Geometry: final body of the model. Coordinates: model frame, mm. A direction names the side the tool comes from. Give positions to 0.01 mm unless a question says otherwise; leave off trailing zeros. Loops run counter-clockwise (first coordinate to the right, second up) from the corner with the lowest first, then second, coordinate; pieces in that order, holes last. Notation, with made-up numbers: (-1, 48) - (22, 48) arc R30 cw to (22, 78) - close; hole circle Ø6 at (21, 56). An arc over 180 degrees is marked (long way). Use CSV: the item, a comma, the result in double quotes. Start each with the question number.
```python
from build123d import *

# Parameters (mm, degrees)
ESBO_O1_R                = 1.5
ESBO_O1_W                = 5
ESBO_O1_H                = 35
RESSALTO_EXTRUS_O1_DEPTH = 3
ESBO_O2_W                = 25
ESBO_O2_H                = 5
RESSALTO_EXTRUS_O2_DEPTH = 15
FILETE5_R                = 5
FILETE6_R                = 5
FILETE7_R                = 5
FILETE8_R                = 5
ESBO_O4_R                = 1
ESBO_O4_W                = 4
ESBO_O4_H                = 4
CORTE_EXTRUS_O2_DEPTH    = 5
CORTE_EXTRUS_O3_START    = -5
ESBO_O3_R                = 1
ESBO_O3_R_2              = 1.5
ESBO_O3_W                = 4
ESBO_O3_H                = 7
CORTE_EXTRUS_O3_DEPTH    = 5


with BuildPart() as part:
    # Esboço1 → Ressalto-extrusão1 (new body)
    with BuildSketch(Plane.XY):
        Polygon((-24.430369357, 7.066666667), (10.569630643, 7.066666667), (10.569630643, 2.066666667), (5.569630643, 2.066666667), (5.569630643, -32.933333333), (10.569630643, -32.933333333), (10.569630643, -37.933333333), (-24.430369357, -37.933333333), (-24.430369357, -32.933333333), (-19.430369357, -32.933333333), (-19.430369357, 2.066666667), (-24.430369357, 2.066666667), align=None)
        with Locations((-14.430369357, -4.933333333)):
            Circle(ESBO_O1_R, mode=Mode.SUBTRACT)
        with Locations((-14.430369357, -11.933333333)):
            Circle(ESBO_O1_R, mode=Mode.SUBTRACT)
        with Locations((-14.430369357, -18.933333333)):
            Circle(ESBO_O1_R, mode=Mode.SUBTRACT)
        with Locations((0.569630643, -4.933333333)):
            Circle(ESBO_O1_R, mode=Mode.SUBTRACT)
        with Locations((0.569630643, -18.933333333)):
            Circle(ESBO_O1_R, mode=Mode.SUBTRACT)
        with Locations((0.569630643, -25.933333333)):
            Circle(ESBO_O1_R, mode=Mode.SUBTRACT)
        with Locations((-14.430369357, -25.933333333)):
            Circle(ESBO_O1_R, mode=Mode.SUBTRACT)
        with Locations((0.569630643, -11.933333333)):
            Circle(ESBO_O1_R, mode=Mode.SUBTRACT)
        with Locations((-21.930369357, 4.566666667)):
            Circle(ESBO_O1_R, mode=Mode.SUBTRACT)
        with Locations((8.069630643, 4.566666667)):
            Circle(ESBO_O1_R, mode=Mode.SUBTRACT)
        with Locations((-21.930369357, -35.433333333)):
            Circle(ESBO_O1_R, mode=Mode.SUBTRACT)
        with Locations((8.069630643, -35.433333333)):
            Circle(ESBO_O1_R, mode=Mode.SUBTRACT)
        with Locations((-6.930369357, -15.433333333)):
            Rectangle(ESBO_O1_W, ESBO_O1_H, mode=Mode.SUBTRACT)
    extrude(amount=-RESSALTO_EXTRUS_O1_DEPTH)

    # Esboço2 → Ressalto-extrusão2 (add)
    with BuildSketch(Plane.XY):
        with Locations((-6.930369357, 4.566666667)):
            Rectangle(ESBO_O2_W, ESBO_O2_H)
        with Locations((-6.930369357, -35.433333333)):
            Rectangle(ESBO_O2_W, ESBO_O2_H)
    extrude(amount=RESSALTO_EXTRUS_O2_DEPTH)

    # Filete5
    filete5_edges = [part.edges().sort_by_distance(p)[0] for p in [
        (5.569630643, -35.433333333, 15),
    ]]
    fillet(filete5_edges, radius=FILETE5_R)

    # Filete6
    filete6_edges = [part.edges().sort_by_distance(p)[0] for p in [
        (-19.430369357, -35.433333333, 15),
    ]]
    fillet(filete6_edges, radius=FILETE6_R)

    # Filete7
    filete7_edges = [part.edges().sort_by_distance(p)[0] for p in [
        (-19.430369357, 4.566666667, 15),
    ]]
    fillet(filete7_edges, radius=FILETE7_R)

    # Filete8
    filete8_edges = [part.edges().sort_by_distance(p)[0] for p in [
        (5.569630643, 4.566666667, 15),
    ]]
    fillet(filete8_edges, radius=FILETE8_R)

    # Esboço4 → Corte-extrusão2 (cut)
    with BuildSketch(Plane(origin=(0, 7.066666667, 0), x_dir=(1, 0, 0), z_dir=(0, 1, 0))):
        with Locations(Location((-13.180369357, -6, 0), (0, 0, 180))):
            Circle(ESBO_O4_R)
        with Locations(Location((-0.680369357, -6, 0), (0, 0, 180))):
            Circle(ESBO_O4_R)
        with Locations((-6.930369357, -6)):
            Rectangle(ESBO_O4_W, ESBO_O4_H)
    extrude(amount=-CORTE_EXTRUS_O2_DEPTH, mode=Mode.SUBTRACT)

    # Esboço3 → Corte-extrusão3 (cut)
    with BuildSketch(Plane(origin=(0, -37.933333333, 0), x_dir=(-1, 0, 0), z_dir=(0, -1, 0)).offset(CORTE_EXTRUS_O3_START)):
        with Locations((13.180369357, -6)):
            Circle(ESBO_O3_R)
        with Locations(Location((0.680369357, -6.000000354, 0), (0, 0, 2.0294e-05))):
            Circle(ESBO_O3_R)
        with Locations(Location((14.430369357, -11.516860689, 0), (0, 0, 180))):
            Circle(ESBO_O3_R_2)
        with Locations(Location((-0.569630643, -11.516860689, 0), (0, 0, 180))):
            Circle(ESBO_O3_R_2)
        with Locations((6.930369357, -4.5)):
            Rectangle(ESBO_O3_W, ESBO_O3_H)
    extrude(amount=CORTE_EXTRUS_O3_DEPTH, mode=Mode.SUBTRACT)


solid = part.part
```
Item 1: Section C-C (z = 6). Give the number of separate pieces and of enclosed holes in the cut face, plus the area to 3 significant figures.
Item 2: Section A-A (z = 3). Output: boundary loops of the cut face in (x, y).
Item 3: Ray query, probe 1 along X at (y, z) = (-2, -1.75); probe 2 along Y at (x, z) = (-11.5, 5.5); probe 3 along Z at (x, y) = (4, -9.5). Return the intervals inside material, ascending.
Item 4: Mould query, pull axis X, two halves, no side actions, for faces 1 (the flat face through (-7, 5, 4)), 2 (the cylindrical face through (4.07, 4.6, 13.57)), 3 (the flat face through (-22, -32.933, -1)). Classes: pulls with the +X half, pulls with the -X half, needs draft (parallel to the pull), parting line crosses it, or undercut.
Item 5: Reachability of faces 4 (the flat face through (5.57, -35, 5)), 5 (the flat face through (-7, -35, 1)), 6 (the flat face through (-4.43, -16, -1)) from +Z, -Z, +X, -X, +Y, -Y: full face, straight path, thin tool, end or side. Return the list, or none.
Item 6: Section B-B (y = -29.5). Output: boundary loops of the cut face in (x, z), plus the area to 3 significant figures.
Item 7: Pin query (flat end, axial travel): pin 1 Ø4 at (x, y) = (-14.43, -18.93) entering from +Z; pin 2 Ø2.5 at (y, z) = (-17.5, -1.5) entering from +X; pin 3 Ø2 at (y, z) = (5.5, 6) entering from -X. Return the tip coordinate at first contact, or that it passes through.
Item 8: Section D-D (y = 4). Output: boundary loops of the cut face in (x, z).
Outcome:
1,separate pieces,"8"
1,enclosed holes,"0"
1,area,"170 mm2"
2,outline,"(-19.43, -37.93) - (-8.93, -37.93) - (-8.93, -32.93) - (-19.43, -32.93) - close; (-19.43, 2.07) - (5.57, 2.07) - (5.57, 7.07) - (-19.43, 7.07) - close; (-4.93, -37.93) - (5.57, -37.93) - (5.57, -32.93) - (-4.93, -32.93) - close"
3,probe 1,"x = -19.43 to -9.43, -4.43 to 5.57"
3,probe 2,"y = -37.93 to -32.93, 2.07 to 7.07"
3,probe 3,"z = -3 to 0"
4,face 1,"undercut"
4,face 2,"pulls with the +X half"
4,face 3,"needs draft"
5,face 4,"+Z, +X, +Y, -Y"
5,face 5,"-Y"
5,face 6,"+Z, -Z"
6,outline,"(-19.43, -3) - (-9.43, -3) - (-9.43, 0) - (-19.43, 0) - close; (-4.43, -3) - (5.57, -3) - (5.57, 0) - (-4.43, 0) - close"
6,area,"60.0 mm2"
7,pin 1,"stops at z = 0"
7,pin 2,"stops at x = 5.57"
7,pin 3,"stops at x = -19.43"
8,outline,"(-24.43, -3) - (-23.32, -3) - (-23.32, 0) - (-24.43, 0) - close; (-20.54, -3) - (6.68, -3) - (6.68, 0) - (5.57, 0) - (5.57, 10) arc R5 ccw to (0.57, 15) - (-14.43, 15) arc R5 ccw to (-19.43, 10) - (-19.43, 0) - (-20.54, 0) - close; (9.46, -3) - (10.57, -3) - (10.57, 0) - (9.46, 0) - close; hole circle Ø2 at (-13.18, 6); hole (-8.93, 4) - (-4.93, 4) - (-4.93, 8) - (-8.93, 8) - close; hole circle Ø2 at (-0.68, 6)"
